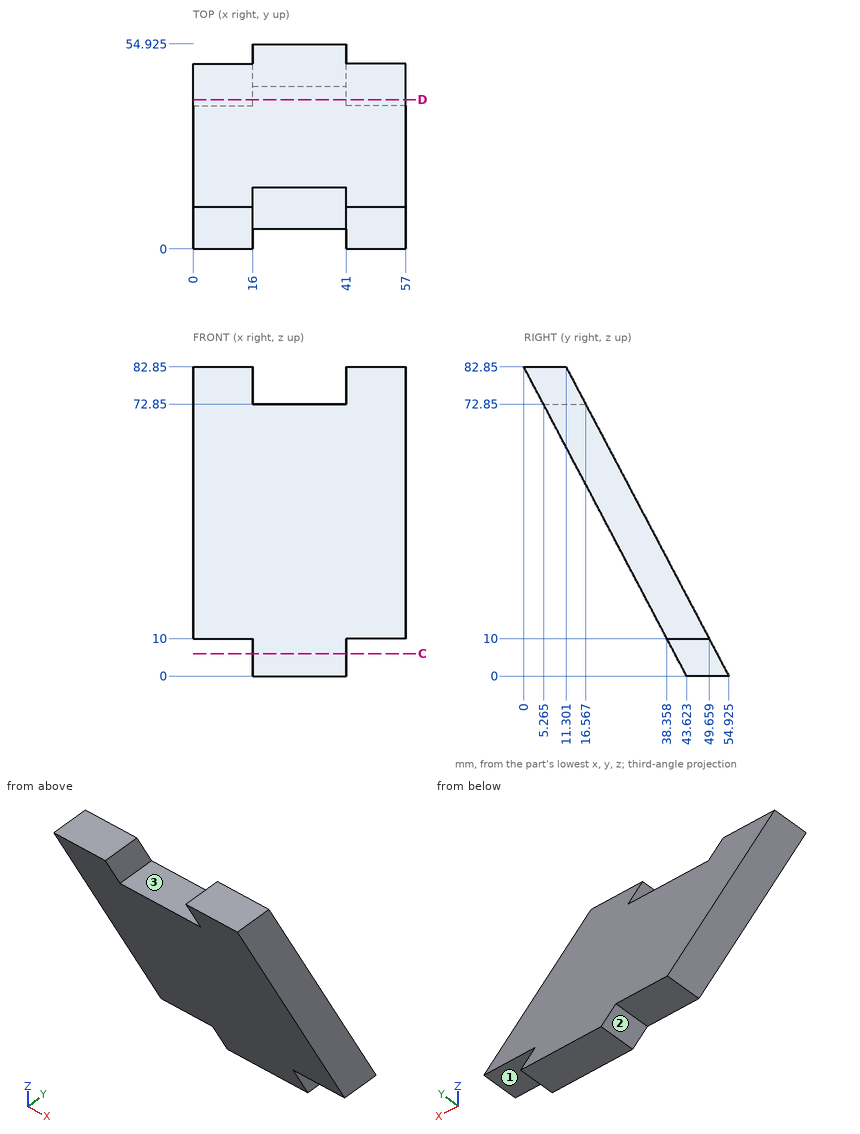
Geometry check sheet. Reference: drawing and pictorial views, mm from the part's lowest x, y, z. A direction names the side the tool comes from. Give positions to 0.01 mm unless a question says otherwise; leave off trailing zeros. Order: outer loops, then holes, each group sorted by start corner. A loop starts at its lowest first (then second) coordinate and runs counter-clockwise, first axis right, second up. Notation, with made-up numbers: M -30,87.5 L 7,87.5 A18 ccw 7,111.5 Z; hole C 72.25,15.25 d4. An arc over 180 degrees is marked long. Answer as a JSON object with one key per item and string values. Group by question number.
1) Cross-section at D-D (y = 40). Enter the section's corners in (x, z) (1 decimal), then the cut area to 3 significant figures.
2) Depth check by flat-ended pin: pin 1 Ø12.5 at (x, y) = (51, 43) entering from -Z; pin 2 Ø3 at (y, z) = (44, 5.5) entering from -X; pin 3 Ø5 at (x, y) = (46, 13.5) entering from +Z; pin 4 Ø9 at (x, y) = (33.5, 11.5) entering from +Z. Enter the tip coordinate at first touch or a pass-through.
3) Access from +Z, -Z, +X, -X, +Y, -Y to the whole of each face (thin tool, end or side, straight path). Record for the marked faces 1, 2 and 3.
4) Cross-section at C-C (z = 6). Enter the section's corners in (x, y) (1 decimal).
5) Scan lines: line 1 along Z through (x, y) = (39.5, 53) (1 decimal); line 2 along Y through (x, z) = (48.5, 65.5) (1 decimal); line 3 along Y through (x, z) = (39, 32) (1 decimal). Record each from-to range of solid material in increasing order. Write a range as [from, to].
Result sheet:
{
 "1": {"outline": "M 0,10 L 16,10 L 16,6.9 L 41,6.9 L 41,10 L 57,10 L 57,28.3 L 0,28.3 Z", "area": "1,120 mm2"},
 "2": {"pin 1": "stops at z = 10", "pin 2": "stops at x = 16", "pin 3": "stops at z = 82.85", "pin 4": "stops at z = 72.85"},
 "3": {"face 1": "-Z, +X, +Y, -Y", "face 2": "-Z, -X, +Y, -Y", "face 3": "+Z, +Y, -Y"},
 "4": {"outline": "M 16,40.5 L 41,40.5 L 41,51.8 L 16,51.8 Z"},
 "5": {"line 1": "z = [0, 3.7]", "line 2": "y = [9.1, 20.4]", "line 3": "y = [26.8, 38.1]"}
}
